The listing builds one solid part. Answer for the finished solid, in the listing's coordinates (mm). A direction names the side the tool comes from. Give positions to 0.01 mm unless a question says otherwise; leave off trailing zeros. Order: outer loops, then holes, each group sorted by start corner. A loop starts at its lowest first (then second) coordinate and runs counter-clockwise, first axis right, second up. Notation, with made-up numbers: (10.25, -10.5) - (20.25, -10.5) arc R11 cw to (20.25, 6.5) - close; hole circle Ø1 at (73.25, -38). An arc over 180 degrees is marked (long way). Answer as CSV lines item,"result". Start each with the question number.
1. Flat-ended cylindrical pins translate along their axes: pin 1 (5 mm diameter, centred on x = -10, z = -11.5, fed in from -Y); pin 2 (2.5 mm diameter, centred on y = -22, z = -14.5, fed in from +X); pin 3 (3 mm diameter, centred on x = -3, y = 6, fed in from -Z); pin 4 (5 mm diameter, centred on y = -16.5, z = -9, fed in from -X). Find the tip coordinate at first contact, or state that the pin passes through.
2. Section A-A on z = -16.5 is taken. Give the vertices of the cut face in (x, y), and give its area (3 significant figures).
3. Section C-C on x = -0.25 is taken. Give the vertices of the cut face in (y, z), and give its area (3 significant figures).
4. Consider line 1 along Y through (x, z) = (5, -4.5); line 2 along Y through (x, z) = (-2.75, -0.75); line 3 along X through (y, z) = (-13, -13.5). Determine where each line is inside the solid, lowest interval first. Write a range as [from, to].
5. Section D-D on x = -3.25 is taken. Give the vertices of the cut face in (y, z), and give its area (3 significant figures).
6. Which of the six approach directions +Z, -Z, +X, -X, +Y, -Y give full straight-line access (tool end or side, diameter ignored) to faces 1 (the flat face through (-2.5, -23, -16)), 2 (the flat face through (-2, 5, -3.929)), 3 (the cylindrical face through (-6.24, -15.14, -13.06))?
7. Section B-B on y = -16 is taken. Give the vertices of the cut face in (x, z).
Autodesk Inventor part; units mm, degrees
ref_plane "YZ Plane" through (0, 0, 0) normal (1, 0, 0) x (0, 1, 0)
ref_plane "XZ Plane" through (0, 0, 0) normal (0, 1, 0) x (-1, 0, 0)
ref_plane "XY Plane" through (0, 0, 0) normal (0, 0, 1) x (1, 0, 0)
sketch "Sketch1" plane through (0, 0, 0) normal (0, 1, 0) x (-1, 0, 0)
  line L0 (0, 0) -> (0, -13)
  line L1 (0, -13) -> (-2, -13)
  line L2 (-2, -13) -> (-2, 2)
  line L3 (-2, 2) -> (12, 2)
  line L4 (12, 2) -> (12, -13)
  line L5 (12, -13) -> (10, -13)
  line L6 (10, -13) -> (10, 0)
  line L7 (10, 0) -> (0, 0)
  dimension "d0" = 13
  dimension "d1" = 2
  dimension "d2" = 15
  dimension "d3" = 14
  dimension "d4" = 2
  dimension "d5" = 13
ref_plane "Work Plane2" through (-12, 0, 2) normal (0, 0, 1) x (1, 0, 0)
sketch "Sketch2" plane through (-12, 0, 2) normal (0, 0, 1) x (1, 0, 0)
  line L0 (0, 20) -> (14, 20)
  line L1 (7, 20) -> (7, 0)
  line L2 (12, 0) -> (2, 0)
  line L3 (7, 0) -> (7, 4.5)
  circle A0 centre (7, 4.5) radius 1.75
  line L4 (7, 4.5) -> (7, 15.5)
  circle A1 centre (7, 15.5) radius 1.75
  dimension "d8" = 4.5
  dimension "d9" = 3.5
  dimension "d10" = 11
  dimension "d11" = 3.5
ref_plane "Work Plane5" through (0, 0, 0) normal (0, -1, 0) x (1, 0, 0)
sketch "Sketch3" plane through (0, 0, 0) normal (0, -1, 0) x (1, 0, 0)
  line L0 (-12, 2) -> (2, 2)
  line L1 (-12, -13) -> (-12, 2)
  line L2 (2, 2) -> (-12, 2)
  line L3 (-12, 2) -> (-12, -13)
  line L4 (-12, -13) -> (2, -13)
  line L5 (2, -13) -> (2, 2)
  point P0 (0, 0)
extrude "Extrusion3" add sketch "Sketch3" along normal blind 5
ref_plane "Work Plane6" through (0, -5, 0) normal (0, -1, 0) x (1, 0, 0)
sketch "Sketch4" plane through (0, -5, 0) normal (0, -1, 0) x (1, 0, 0)
  line L0 (-12, -13) -> (2, -13)
  line L1 (2, -13) -> (-12, -13)
  line L2 (-12, -13) -> (-12, -8)
  line L3 (-12, -8) -> (2, -8)
  line L4 (2, -8) -> (2, -13)
  point P0 (0, 0)
  dimension "d16" = 14
  dimension "d17" = 5
ref_plane "Work Plane1" through (0, -25, 0) normal (0, -1, 0) x (1, 0, 0)
sketch "Sketch5" plane through (0, -25, 0) normal (0, -1, 0) x (1, 0, 0)
  line L0 (2, -8) -> (2, -13)
  line L1 (-12, -13) -> (2, -13)
  line L2 (-5, -13) -> (-5, 2)
  line L3 (2, 2) -> (-12, 2)
  line L4 (-5, -13) -> (-2.5, -13)
  line L5 (-10, -13) -> (0, -13)
  line L6 (-2.5, -13) -> (-2.5, -18)
  line L7 (-2.5, -18) -> (-7.5, -18)
  line L8 (-7.5, -18) -> (-7.5, -13)
  line L9 (-2.5, -13) -> (-7.5, -13)
  line L10 (-5, -13) -> (-5, -25.5)
  arc A0 (-2.4988, -13.2528) -> (-5, -13) centre (-5, -25.5) ccw
  arc A1 (-5, -13) -> (-7.5, -13.2526) centre (-5, -25.5) ccw
  point P0 (0, 0)
  point P1 (-2.5, -13.2526)
  dimension "d25" = 2.5
  dimension "d26" = 5
  dimension "d27" = 5
  dimension "d31" = 12.5
extrude "Extrusion4" add sketch "Sketch5" against normal blind 20 contours A0 L6 L7 L10 | L10 L7 L8 A1
ref_plane "Work Plane3" through (2, 20, -13) normal (0, 0, -1) x (-1, 0, 0)
sketch "Sketch6" plane through (2, 20, -13) normal (0, 0, -1) x (-1, 0, 0)
  line L0 (0, -25) -> (0, 0)
  line L1 (14, -25) -> (7, -25)
  line L2 (0, -20) -> (14, -20)
  line L3 (14, -20) -> (14, -25)
  line L4 (14, -25) -> (0, -25)
  line L5 (0, -25) -> (0, -20)
  point P0 (2, -20)
  point P1 (9.5, -25)
  point P2 (9.5, -25)
extrude "Extrusion5" add sketch "Sketch6" along normal up to surface (5 mm away)
ref_plane "Work Plane4" through (-10, 20, -13) normal (0, 0, -1) x (-1, 0, 0)
sketch "Sketch9" plane through (0, -25, 0) normal (0, -1, 0) x (1, 0, 0)
  arc A0 (-2.5, -13.2526) -> (-7.5, -13.2526) centre (-5, -25.5) ccw
  line L0 (-7.5, -13.2526) -> (-7.5, -18)
  line L1 (-7.5, -18) -> (-2.5, -18)
  line L2 (-2.5, -18) -> (-2.5, -13.2526)
  line L3 (-2.5, -18) -> (-2.5, -13.2526)
  line L4 (-2.5, -11.2171) -> (-2.5, -18)
  line L5 (-2.5, -18) -> (-7.5, -18)
  line L6 (2, -18) -> (-12, -18)
  line L7 (-7.5, -18) -> (-7.5, -13.2526)
  point P0 (0, 0)
extrude "Extrusion7" add sketch "Sketch9" along normal blind 15
sketch "Sketch11" plane through (2, 0, -18) normal (0, 0, -1) x (-1, 0, 0)
  line L0 (9.5, -5) -> (9.5, -40)
  line L1 (14, -5) -> (9.5, -5)
  line L2 (14, 0) -> (14, -5)
  line L3 (0, 0) -> (14, 0)
  line L4 (0, -5) -> (0, 0)
  line L5 (4.5, -5) -> (0, -5)
  line L6 (4.5, -5) -> (4.5, -40)
  line L7 (9.5, -40) -> (4.5, -40)
  line L8 (9.5, -5) -> (4.5, -5)
  line L9 (0, -5) -> (14, -5)
  line L10 (0, -5) -> (-5, -5)
  line L11 (-5, -5) -> (-5, 0)
  line L12 (0, -5) -> (0, 0)
  line L13 (-5, 0) -> (0, 0)
  line L14 (14, -5) -> (19, -5)
  line L15 (19, -5) -> (19, 0)
  line L16 (19, 0) -> (14, 0)
  point P0 (2, 0)
  dimension "d39" = 5
  dimension "d40" = 5
extrude "Extrusion9" add sketch "Sketch11" against normal up to surface (20 mm away) contours L10 L11 L13 L4
sketch "Sketch12" plane through (7, -5, -18) normal (1, 0, 0) x (0, 0, -1)
  line L0 (-14.0041, 5.1427) -> (-14.0041, 5) construction
  line L1 (-20, 5) -> (0, 5) construction
  line L2 (-14.0041, 5) -> (-18.0041, 5) construction
  line L3 (-20, 0) -> (0, 0)
  line L4 (-18.0041, 5) -> (-20, 5)
  line L5 (-20, 5) -> (-20, 0)
  line L6 (-20, 0) -> (-18.0041, 0)
  line L7 (-18.0041, 0) -> (-18.0041, 5)
  point P0 (-18, 5)
  dimension "d43" = 4
extrude "Extrusion10" cut sketch "Sketch12" against normal through all
sketch "Sketch13" plane through (7, -5, -18) normal (1, 0, 0) x (0, 0, -1)
  line L0 (0, 5) -> (-18.0041, 5)
  line L1 (-18.0041, 5) -> (-14.0707, 5)
  line L2 (-14.0707, 5) -> (-14.0707, 15.1381)
  line L3 (-14.0707, 15.1381) -> (-18.0041, 15.1381)
  line L4 (-18.0041, 15.1381) -> (-18.0041, 5)
  point P0 (-18, 5)
extrude "Extrusion11" add sketch "Sketch13" against normal up to surface (19 mm away)
equation "\"d41\" = d40"
Checks:
1,pin 1,"stops at y = -5"
1,pin 2,"stops at x = -2.5"
1,pin 3,"stops at z = -3.93"
1,pin 4,"passes through"
2,outline,"(-12, -5) - (-7.5, -5) - (-7.5, -40) - (-2.5, -40) - (-2.5, -5) - (7, -5) - (7, 0) - (-12, 0) - close"
2,area,"270 mm²"
3,outline,"(-5, -18) - (0, -18) - (0, -3.93) - (10.14, -3.93) - (10.14, 0) - (-5, 0) - close"
3,area,"130 mm²"
4,line 1,"y = [-5, 0]"
4,line 2,"y = [-5, 10.14]"
4,line 3,"x = [-7.5, -2.5]"
5,outline,"(-40, -18) - (0, -18) - (0, -3.93) - (10.14, -3.93) - (10.14, 0) - (-5, 0) - (-5, -13.12) - (-40, -13.12) - close"
5,area,"301 mm²"
6,face 1,"+Z, -Z, +X, -Y"
6,face 2,"-Z, +X, -X, +Y"
6,face 3,"+Z, -X, -Y"
7,outline,"(-7.5, -18) - (-2.5, -18) - (-2.5, -13.25) arc R12.5 ccw to (-5, -13) arc R12.5 ccw to (-7.5, -13.25) - close"
